Design review of the part built by this model. Coordinates are the model's own, in mm. Face numbers are marked on the shaded views. Give positions to 0.01 mm unless a question says otherwise; leave off trailing zeros. Loops run counter-clockwise (first coordinate to the right, second up) from the corner with the lowest first, then second, coordinate; pieces in that order, holes last.
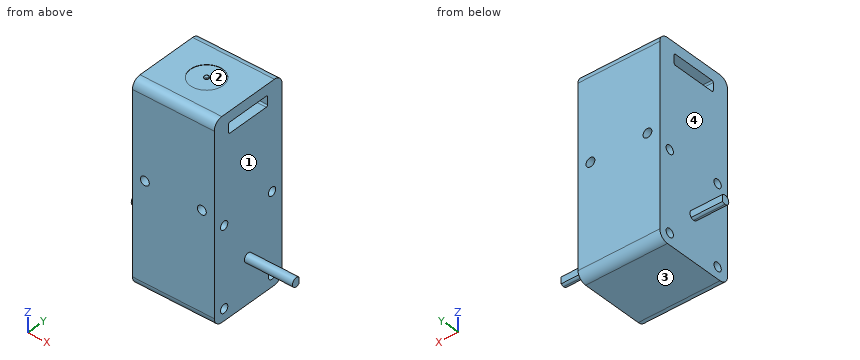
from build123d import *

# Parameters (mm, degrees)
SKETCH1_R           = 1.45
BOSS_EXTRUDE1_DEPTH = 27.7
FILLET1_R           = 3
FILLET2_R           = 0.5
SKETCH2_R           = 1.5
CUT_EXTRUDE1_DEPTH  = 27.7
BOSS_EXTRUDE2_DEPTH = 10.6
BOSS_EXTRUDE3_DEPTH = 44
SKETCH4_R           = 7.25
BOSS_EXTRUDE4_DEPTH = 19
SKETCH5_R           = 5.5
CUT_EXTRUDE2_DEPTH  = 0.1
SKETCH6_R           = 0.75
BOSS_EXTRUDE6_DEPTH = 0.4
FILLET3_R           = 0.2


with BuildPart() as part:
    # Sketch1 → Boss-Extrude1 (new body)
    # profile 1 of 2: a face of its own
    with BuildSketch(Plane(origin=(0, 0, 0), x_dir=(0, 0, -1), z_dir=(1, 0, 0))):
        with BuildLine():
            Line((-39.103654485, -4.271617427), (-42.703654485, -4.271617427))
            Line((-42.703654485, -4.271617427), (-42.703654485, -17.771617427))
            Line((-42.703654485, -17.771617427), (23.896345515, -17.771617427))
            Line((23.896345515, -17.771617427), (23.896345515, -4.271617427))
            Line((23.896345515, -4.271617427), (10.396345515, -4.271617427))
            ThreePointArc((10.396345515, -4.271617427), (8.896345515, -5.771617427), (7.396345515, -4.271617427))
            Line((7.396345515, -4.271617427), (-35.503654485, -4.271617427))
            Line((-35.503654485, -4.271617427), (-35.503654485, -12.071617427))
            Line((-35.503654485, -12.071617427), (-39.103654485, -12.071617427))
            Line((-39.103654485, -12.071617427), (-39.103654485, -4.271617427))
        make_face()
        with Locations((-6.953654485, -13.821617427)):
            Circle(SKETCH1_R, mode=Mode.SUBTRACT)
        with Locations((19.946345515, -13.821617427)):
            Circle(SKETCH1_R, mode=Mode.SUBTRACT)
    # profile 2 of 2: a face of its own
    with BuildSketch(Plane(origin=(0, 0, 0), x_dir=(0, 0, -1), z_dir=(1, 0, 0))):
        with BuildLine():
            Line((-42.703654485, 9.228382573), (-42.703654485, -4.271617427))
            Line((-42.703654485, -4.271617427), (-39.103654485, -4.271617427))
            Line((-39.103654485, -4.271617427), (-39.103654485, 3.528382573))
            Line((-39.103654485, 3.528382573), (-35.503654485, 3.528382573))
            Line((-35.503654485, 3.528382573), (-35.503654485, -4.271617427))
            Line((-35.503654485, -4.271617427), (7.396345515, -4.271617427))
            ThreePointArc((7.396345515, -4.271617427), (8.896345515, -2.771617427), (10.396345515, -4.271617427))
            Line((10.396345515, -4.271617427), (23.896345515, -4.271617427))
            Line((23.896345515, -4.271617427), (23.896345515, 9.228382573))
            Line((23.896345515, 9.228382573), (-42.703654485, 9.228382573))
        make_face()
        with Locations((-6.953654485, 5.278382573)):
            Circle(SKETCH1_R, mode=Mode.SUBTRACT)
        with Locations((19.946345515, 5.278382573)):
            Circle(SKETCH1_R, mode=Mode.SUBTRACT)
    extrude(amount=BOSS_EXTRUDE1_DEPTH)

    # Fillet1
    fillet1_edges = [part.edges().sort_by_distance(p)[0] for p in [
        (13.85, -17.771617427, -23.896345515),
        (13.85, -17.771617427, 42.703654485),
        (13.85, 9.228382573, 42.703654485),
        (13.85, 9.228382573, -23.896345515),
    ]]
    fillet(fillet1_edges, radius=FILLET1_R)

    # Fillet2
    fillet2_edges = [part.edges().sort_by_distance(p)[0] for p in [
        (13.85, -12.071617427, 39.103654485),
        (13.85, -12.071617427, 35.503654485),
        (13.85, 3.528382573, 35.503654485),
        (13.85, 3.528382573, 39.103654485),
    ]]
    fillet(fillet2_edges, radius=FILLET2_R)

    # Sketch2 → Cut-Extrude1 (cut)
    with BuildSketch(Plane(origin=(0, 9.228382573, 0), x_dir=(1, 0, 0), z_dir=(0, 1, 0))):
        with Locations(Location((4.2, -12.103654485, 0), (0, 0, 270))):
            Circle(SKETCH2_R)
        with Locations(Location((23.5, -12.103654485, 0), (0, 0, 270))):
            Circle(SKETCH2_R)
    extrude(amount=-CUT_EXTRUDE1_DEPTH, mode=Mode.SUBTRACT)



with BuildPart() as body_2:
    # Sketch3 → Boss-Extrude2 (new body)
    with BuildSketch(Plane(origin=(0, 0, 0), x_dir=(0, 0, -1), z_dir=(1, 0, 0))):
        with BuildLine():
            Line((10.014379504, -3.271617427), (7.778311526, -3.271617427))
            ThreePointArc((7.778311526, -3.271617427), (8.36111238, -5.672875965), (10.396345515, -4.271617427))
            ThreePointArc((10.396345515, -4.271617427), (10.297604053, -3.736384292), (10.014379504, -3.271617427))
        make_face()
    extrude(amount=-BOSS_EXTRUDE2_DEPTH)


with BuildPart() as part_1:
    add(part.part)

    add(body_2.part)  # Boss-Extrude3 merges body 2
    # Sketch3_4 → Boss-Extrude3 (add)
    with BuildSketch(Plane(origin=(0, 0, 0), x_dir=(0, 0, -1), z_dir=(1, 0, 0))):
        with BuildLine():
            Line((10.014379504, -3.271617427), (7.778311526, -3.271617427))
            ThreePointArc((7.778311526, -3.271617427), (8.36111238, -5.672875965), (10.396345515, -4.271617427))
            ThreePointArc((10.396345515, -4.271617427), (10.297604053, -3.736384292), (10.014379504, -3.271617427))
        make_face()
    extrude(amount=BOSS_EXTRUDE3_DEPTH)

    # Sketch4 → Boss-Extrude4 (add)
    with BuildSketch(Plane(origin=(0, 0, 39.103654485), x_dir=(-1, 0, 0), z_dir=(0, 0, -1))):
        with Locations((-13.85, -4.271617427)):
            Circle(SKETCH4_R)
    extrude(amount=BOSS_EXTRUDE4_DEPTH)

    # Sketch5 → Cut-Extrude2 (cut)
    with BuildSketch(Plane.XY.offset(42.703654485)):
        with Locations((13.85, -4.521617427)):
            Circle(SKETCH5_R)
    extrude(amount=-CUT_EXTRUDE2_DEPTH, mode=Mode.SUBTRACT)

    # Sketch6 → Boss-Extrude6 (add)
    with BuildSketch(Plane.XY.offset(42.603654485)):
        with Locations((13.85, -4.521617427)):
            Circle(SKETCH6_R)
    extrude(amount=BOSS_EXTRUDE6_DEPTH)

    # Fillet3
    fillet3_edges = [part_1.edges().sort_by_distance(p)[0] for p in [
        (13.1, -4.521617427, 43.003654485),
    ]]
    fillet(fillet3_edges, radius=FILLET3_R)


solid = part_1.part
Q1. Draft analysis for pull direction X (two halves, no side actions). For the marked faces 1, 2, 3 and 4, state which applies: pulls with the +X half, pulls with the -X half, needs draft (parallel to the pull), parting line crosses it, or undercut.
Results:
face 1: pulls with the +X half
face 2: undercut
face 3: needs draft
face 4: pulls with the -X half
Q2. Take a section at B-B (x = 10.5). Give the number of separate pieces and of enclosed holes in the cut face, plus the area to 3 significant figures.
Results:
separate pieces: 1
enclosed holes: 7
area: 1,750 mm2
Q3. Wall thickness on line 1 (Z direction, x = 15, y = 5.25); line 2 (Z direction, x = 24, y = 6.5); line 3 (Y direction, x = 3, z = 37.5): over which ranges is each line inside the solid? List them lowest first.
Results:
line 1: z = -23.9 to -21.4, -18.5 to 5.5, 8.4 to 42.7
line 2: z = -23.88 to -20.73, -19.17 to 6.17, 7.73 to 10.69, 13.52 to 42.69
line 3: y = -17.77 to -12.07, 3.53 to 9.23
Q4. Take a section at C-C (z = -16). Give the boundary of the cut face in (x, y).
Results:
outline: (0, -17.77) - (27.7, -17.77) - (27.7, 9.23) - (0, 9.23) - close
Q5. Insertion check: pin 1 (2.5 mm diameter, centred on y = -13.82, z = 6.95, fed in from +X); pin 2 (8 mm diameter, centred on y = -3.5, z = 17, fed in from -X); pin 3 (12 mm diameter, centred on x = 26, y = -13, fed in from +Z); pin 4 (2 mm diameter, centred on y = -1.5, z = 1.5, fed in from +X). Each pin has a flat end and moves straight along its axis. Give the tip position at first contact, or say it passes through.
Results:
pin 1: passes through
pin 2: stops at x = 0
pin 3: stops at z = 42.7
pin 4: stops at x = 27.7
Q6. Take a section at A-A (x = 4.2). Give the boundary of the cut face in (y, z).
Results:
outline: (-17.77, -20.9) arc R3 ccw to (-14.77, -23.9) - (6.23, -23.9) arc R3 ccw to (9.23, -20.9) - (9.23, 10.6) - (-17.77, 10.6) - close; (-17.77, 13.6) - (9.23, 13.6) - (9.23, 39.7) arc R3 ccw to (6.23, 42.7) - (-14.77, 42.7) arc R3 ccw to (-17.77, 39.7) - close; hole circle Ø2.9 at (-13.82, -19.95); hole circle Ø2.9 at (-13.82, 6.95); hole (-12.07, 36) arc R0.5 ccw to (-11.57, 35.5) - (3.03, 35.5) arc R0.5 ccw to (3.53, 36) - (3.53, 38.6) arc R0.5 ccw to (3.03, 39.1) - (-11.57, 39.1) arc R0.5 ccw to (-12.07, 38.6) - close; hole (-3.27, -10.01) arc R1.5 ccw to (-3.27, -7.78) - close; hole circle Ø2.9 at (5.28, -19.95); hole circle Ø2.9 at (5.28, 6.95)
